```python
from build123d import *

# Parameters (mm, degrees)
SKETCH1_W           = 50.8
SKETCH1_H           = 25.4
SKETCH1_W_2         = 45.72
SKETCH1_H_2         = 20.32
BOSS_EXTRUDE1_DEPTH = 171.45
SKETCH2_R           = 2.032
CUT_EXTRUDE1_DEPTH  = 180.268046511
SKETCH3_R           = 2.032
CUT_EXTRUDE2_DEPTH  = 176.172550646


with BuildPart() as part:
    # Sketch1 → Boss-Extrude1 (new, symmetric)
    with BuildSketch(Plane(origin=(0, 0, 0), x_dir=(0, 0, -1), z_dir=(1, 0, 0))):
        Rectangle(SKETCH1_W, SKETCH1_H)
        Rectangle(SKETCH1_W_2, SKETCH1_H_2, mode=Mode.SUBTRACT)
    extrude(amount=BOSS_EXTRUDE1_DEPTH, both=True)

    # Sketch2 → Cut-Extrude1 (cut, through all)
    with BuildSketch(Plane.XY.offset(25.4)):
        with Locations((-171.45, 0)):
            Circle(SKETCH2_R)
        with Locations((-158.75, 0)):
            Circle(SKETCH2_R)
        with Locations((-146.05, 0)):
            Circle(SKETCH2_R)
        with Locations((-133.35, 0)):
            Circle(SKETCH2_R)
        with Locations((-120.65, 0)):
            Circle(SKETCH2_R)
        with Locations((-107.95, 0)):
            Circle(SKETCH2_R)
        with Locations((-95.25, 0)):
            Circle(SKETCH2_R)
        with Locations((-82.55, 0)):
            Circle(SKETCH2_R)
        with Locations((-69.85, 0)):
            Circle(SKETCH2_R)
        with Locations((-57.15, 0)):
            Circle(SKETCH2_R)
        with Locations((-44.45, 0)):
            Circle(SKETCH2_R)
        with Locations((-31.75, 0)):
            Circle(SKETCH2_R)
        with Locations((-19.05, 0)):
            Circle(SKETCH2_R)
        with Locations((-6.35, 0)):
            Circle(SKETCH2_R)
        with Locations((6.35, 0)):
            Circle(SKETCH2_R)
        with Locations((19.05, 0)):
            Circle(SKETCH2_R)
        with Locations((31.75, 0)):
            Circle(SKETCH2_R)
        with Locations((44.45, 0)):
            Circle(SKETCH2_R)
        with Locations((57.15, 0)):
            Circle(SKETCH2_R)
        with Locations((69.85, 0)):
            Circle(SKETCH2_R)
        with Locations((82.55, 0)):
            Circle(SKETCH2_R)
        with Locations((95.25, 0)):
            Circle(SKETCH2_R)
        with Locations((107.95, 0)):
            Circle(SKETCH2_R)
        with Locations((120.65, 0)):
            Circle(SKETCH2_R)
        with Locations((133.35, 0)):
            Circle(SKETCH2_R)
        with Locations((146.05, 0)):
            Circle(SKETCH2_R)
        with Locations((158.75, 0)):
            Circle(SKETCH2_R)
        with Locations((171.45, 0)):
            Circle(SKETCH2_R)
        with Locations((184.15, 0)):
            Circle(SKETCH2_R)
        with Locations((196.85, 0)):
            Circle(SKETCH2_R)
        with Locations((209.55, 0)):
            Circle(SKETCH2_R)
        with Locations((222.25, 0)):
            Circle(SKETCH2_R)
        with Locations((234.95, 0)):
            Circle(SKETCH2_R)
        with Locations((247.65, 0)):
            Circle(SKETCH2_R)
        with Locations((260.35, 0)):
            Circle(SKETCH2_R)
        with Locations((273.05, 0)):
            Circle(SKETCH2_R)
        with Locations((285.75, 0)):
            Circle(SKETCH2_R)
        with Locations((298.45, 0)):
            Circle(SKETCH2_R)
        with Locations((311.15, 0)):
            Circle(SKETCH2_R)
        with Locations((323.85, 0)):
            Circle(SKETCH2_R)
    extrude(amount=-CUT_EXTRUDE1_DEPTH, mode=Mode.SUBTRACT)

    # Sketch3 → Cut-Extrude2 (cut, through all)
    with BuildSketch(Plane.XZ.offset(12.7)):
        with Locations(Location((44.45, 12.7, 0), (0, 0, 270))):
            Circle(SKETCH3_R)
        with Locations(Location((44.45, -12.7, 0), (0, 0, 270))):
            Circle(SKETCH3_R)
        with Locations(Location((-44.45, -12.7, 0), (0, 0, 270))):
            Circle(SKETCH3_R)
        with Locations(Location((-44.45, 12.7, 0), (0, 0, 270))):
            Circle(SKETCH3_R)
    extrude(amount=-CUT_EXTRUDE2_DEPTH, mode=Mode.SUBTRACT)


solid = part.part
```
CAD build for the part. Positions are in the model's coordinates, mm. A direction names the side the tool comes from. Round coordinates to 2 decimals unless told otherwise and drop trailing zeros. Order: outer loops, then holes, each group sorted by start corner. A loop starts at its lowest first (then second) coordinate and runs counter-clockwise, first axis right, second up.
Item 1: Tool access for faces 1 (the face through (2, 10.16, 0)), 2 (the face through (2, 0, 25.4)): list every direction of +Z, -Z, +X, -X, +Y, -Y with a clear straight run to the whole face (end or side of a thin tool).
Item 2: Saw through at C-C on y = 5.5. Write the cut outline in (x, z), then the cut area to 3 significant figures.
Item 3: Probe line 1 along Y through (x, z) = (31.75, 24.15); line 2 along Z through (x, y) = (31, -5); line 3 along Y through (x, z) = (142, 8). List the from-to ranges inside material, lowest first.
Item 4: Saw through at B-B on x = 102. Write the cut outline in (y, z).
Item 5: Mould opens along Y. For faces 3 (the face through (171.45, -11, 0)), 4 (the face through (2, 0, -22.86)), 5 (the face through (2, -12.7, 0)) say: pulls with the +Y half, pulls with the -Y half, needs draft (parallel to the pull), parting line crosses it, or undercut.
Item 6: Saw through at A-A on z = 1. Write the cut outline in (x, y).
Reported:
1. face 1: +X, -X
1. face 2: +Z, +X, -X, +Y, -Y
2. outline: (-171.45, -25.4) - (171.45, -25.4) - (171.45, -22.86) - (-171.45, -22.86) - close; (-171.45, 22.86) - (171.45, 22.86) - (171.45, 25.4) - (-171.45, 25.4) - close
2. area: 1,740 mm2
3. line 1: y = -12.7 to -2.03, 2.03 to 12.7
3. line 2: z = -25.4 to -22.86, 22.86 to 25.4
3. line 3: y = -12.7 to -10.16, 10.16 to 12.7
4. outline: (-12.7, -25.4) - (12.7, -25.4) - (12.7, 25.4) - (-12.7, 25.4) - close; hole (-10.16, -22.86) - (10.16, -22.86) - (10.16, 22.86) - (-10.16, 22.86) - close
5. face 3: needs draft
5. face 4: undercut
5. face 5: pulls with the -Y half
6. outline: (-171.45, -12.7) - (171.45, -12.7) - (171.45, -10.16) - (-171.45, -10.16) - close; (-171.45, 10.16) - (171.45, 10.16) - (171.45, 12.7) - (-171.45, 12.7) - close
